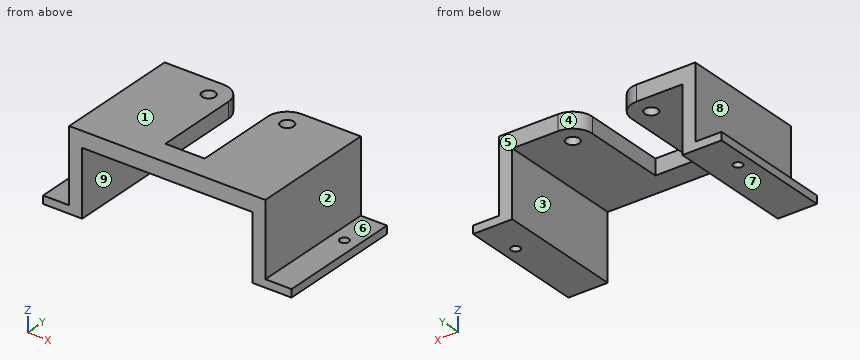
from build123d import *

# Parameters (mm, degrees)
SKETCH107_R   = 2.5
PAD038_DEPTH  = 6
SKETCH108_W   = 5
SKETCH108_H   = 48.5
PAD039_DEPTH  = 22
SKETCH109_W   = 15
SKETCH109_H   = 48.5
PAD040_DEPTH  = 3
SKETCH110_R   = 1.7
HOLE002_DEPTH = 25


with BuildPart() as part:
    # Sketch107 → Pad038 (new body)
    with BuildSketch(Plane.XY.offset(20)):
        with BuildLine():
            Line((-7.5, 7.5), (-7.5, -24.5))
            Line((-7.5, -24.5), (7.5, -24.5))
            Line((7.5, -24.5), (7.5, 7.5))
            ThreePointArc((15, 15), (9.696699, 12.803301), (7.5, 7.5))
            Line((15, 15), (37.5, 15))
            Line((37.5, 15), (37.5, -33.5))
            Line((0, -33.5), (37.5, -33.5))
            Line((-37.5, -33.5), (0, -33.5))
            Line((-37.5, -33.5), (-37.5, 15))
            Line((-37.5, 15), (-15, 15))
            ThreePointArc((-7.5, 7.5), (-9.696699, 12.803301), (-15, 15))
        make_face()
        with Locations((-15, 7.5)):
            Circle(SKETCH107_R, mode=Mode.SUBTRACT)
        with Locations((15, 7.5)):
            Circle(SKETCH107_R, mode=Mode.SUBTRACT)
    extrude(amount=PAD038_DEPTH)

    # Sketch108 → Pad039 (join)
    with BuildSketch(Plane.XY.offset(-2)):
        with Locations((-35, -9.25)):
            Rectangle(SKETCH108_W, SKETCH108_H)
        with Locations((35, -9.25)):
            Rectangle(SKETCH108_W, SKETCH108_H)
    extrude(amount=PAD039_DEPTH)

    # Sketch109 → Pad040 (join)
    with BuildSketch(Plane.XY.offset(-5)):
        with Locations((-40, -9.25)):
            Rectangle(SKETCH109_W, SKETCH109_H)
        with Locations((40, -9.25)):
            Rectangle(SKETCH109_W, SKETCH109_H)
    extrude(amount=PAD040_DEPTH)

    # Sketch110 → Hole002 (cut)
    with BuildSketch(Plane.XY.offset(3)):
        with Locations((-42.5, 0)):
            Circle(SKETCH110_R)
        with Locations((42.5, 0)):
            Circle(SKETCH110_R)
    extrude(amount=-HOLE002_DEPTH, mode=Mode.SUBTRACT)


solid = part.part
Work out the finished part from the listing and answer in its coordinate system (mm). Face numbers are marked on the shaded views. A direction names the side the tool comes from. Round coordinates to 2 decimals unless told otherwise and drop trailing zeros. Write each loop counter-clockwise with the first axis right and the second up, starting at its lowest first coordinate (ties: lowest second). Pieces come first, ordered by that corner, then holes. Notation, with made-up numbers: (79, -17.75) - (110, -17.75) arc R20 ccw to (110, 10.25) - close; hole circle Ø8 at (51.25, 4). An arc over 180 degrees is marked (long way). Answer in a Markdown table with one row per item. Add a question column.
1. A cutting plane is placed at A-A, the plane y = 6. Determine the outline of the cut face in (x, z), and give its area (3 significant figures).
2. A cutting plane is placed at C-C, the plane z = 7. Determine the outline of the cut face in (x, y), and give its area (3 significant figures).
3. The mould has two halves that part along X. Classify the marked faces 1, 2, 3 and 4: +X half, -X half, draft (parallel to the pull), parting line (faces both ways), or undercut.
4. Find the intervals of material crossed by line 1 along X through (y, z) = (8, 10.5); line 2 along Y through (x, z) = (-15, 21.9); line 3 along Y through (x, z) = (42.5, -3.4), in increasing order. Write a range as from..to.
5. A cutting plane is placed at D-D, the plane y = 0. Determine the outline of the cut face in (x, z).
6. Given pin 1 (4.5 mm diameter, centred on x = -42.5, y = 0, fed in from -Z); pin 2 (24.5 mm diameter, centred on x = 7, y = -11.5, fed in from -Z); pin 3 (12 mm diameter, centred on y = 5, z = 12.5, fed in from +X); pin 4 (1.8 mm diameter, centred on y = -15, z = 24, fed in from -X), each flat-ended and moving along its own axis, determine where each tip first touches the part or whether it passes through.
7. A cutting plane is placed at B-B, the plane x = -42.5. Determine the outline of the cut face in (y, z).
8. For the marked faces 5, 6, 7, 8 and 9, determine the directions among +Z, -Z, +X, -X, +Y, -Y from which every point of the face is accessible in a straight line to the end or side of a thin tool.
Worked out:
| question | item | result |
|---|---|---|
| 1 | outline | (-47.5, -5) - (-32.5, -5) - (-32.5, 20) - (-17, 20) - (-17, 26) - (-37.5, 26) - (-37.5, -2) - (-47.5, -2) - close; (-13, 20) - (-7.5, 20) - (-7.5, 26) - (-13, 26) - close; (7.5, 20) - (13, 20) - (13, 26) - (7.5, 26) - close; (17, 20) - (32.5, 20) - (32.5, -5) - (47.5, -5) - (47.5, -2) - (37.5, -2) - (37.5, 26) - (17, 26) - close |
| 1 | area | 622 mm^2 |
| 2 | outline | (-37.5, -33.5) - (-32.5, -33.5) - (-32.5, 15) - (-37.5, 15) - close; (32.5, -33.5) - (37.5, -33.5) - (37.5, 15) - (32.5, 15) - close |
| 2 | area | 485 mm^2 |
| 3 | face 1 | draft |
| 3 | face 2 | +X half |
| 3 | face 3 | undercut |
| 3 | face 4 | undercut |
| 4 | line 1 | -37.5..-32.5, 32.5..37.5 |
| 4 | line 2 | -33.5..5, 10..15 |
| 4 | line 3 | -33.5..-1.7, 1.7..15 |
| 5 | outline | (-47.5, -5) - (-44.2, -5) - (-44.2, -2) - (-47.5, -2) - close; (-40.8, -5) - (-32.5, -5) - (-32.5, 20) - (-7.5, 20) - (-7.5, 26) - (-37.5, 26) - (-37.5, -2) - (-40.8, -2) - close; (7.5, 20) - (32.5, 20) - (32.5, -5) - (40.8, -5) - (40.8, -2) - (37.5, -2) - (37.5, 26) - (7.5, 26) - close; (44.2, -5) - (47.5, -5) - (47.5, -2) - (44.2, -2) - close |
| 6 | pin 1 | z = -5 |
| 6 | pin 2 | z = 20 |
| 6 | pin 3 | x = 37.5 |
| 6 | pin 4 | x = -37.5 |
| 7 | outline | (-33.5, -5) - (-1.7, -5) - (-1.7, -2) - (-33.5, -2) - close; (1.7, -5) - (15, -5) - (15, -2) - (1.7, -2) - close |
| 8 | face 5 | +Z, -Z, +X, -X, +Y |
| 8 | face 6 | +Z, +X, +Y, -Y |
| 8 | face 7 | -Z, +X, -X, +Y, -Y |
| 8 | face 8 | +Z, -X, +Y, -Y |
| 8 | face 9 | -Z, +Y, -Y |
